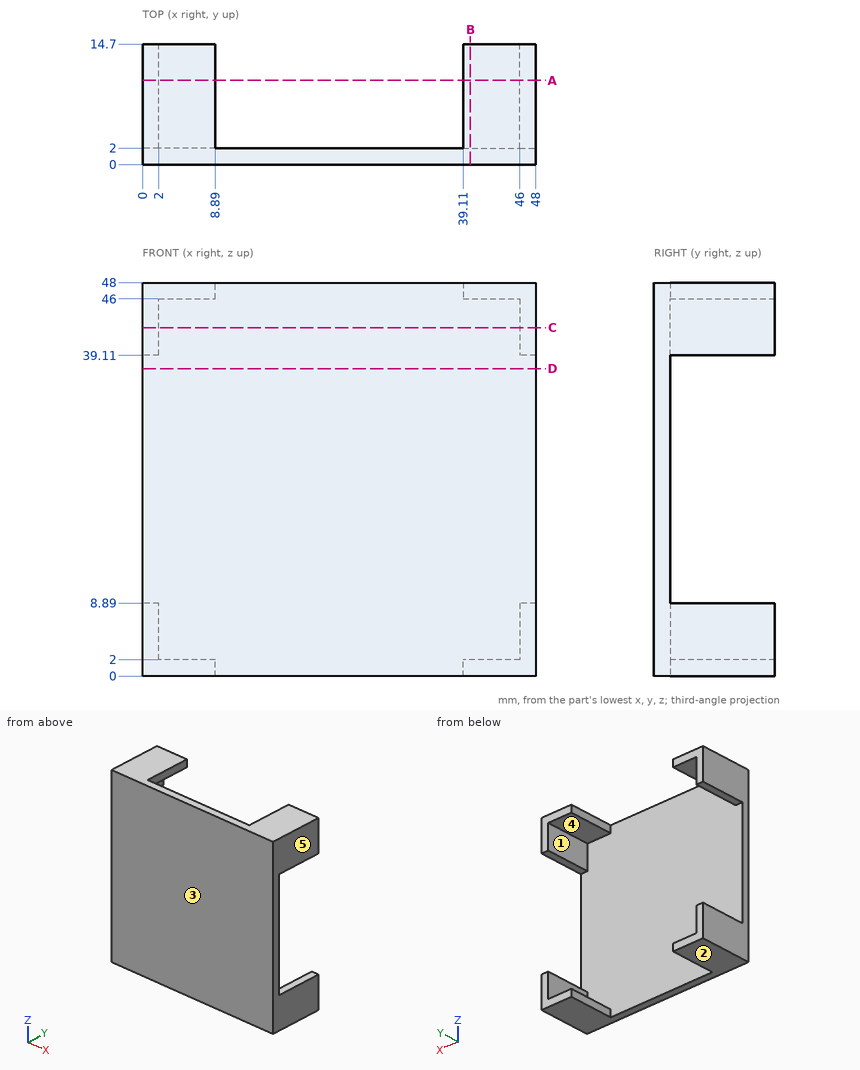
For this review, use the dimensioned drawing (mm, ordinates from the lowest corner) and the shaded views. A direction names the side the tool comes from. Coordinates: 2 decimals unless noted, no trailing zeros. Write each loop counter-clockwise with the first axis right and the second up, starting at its lowest first coordinate (ties: lowest second). Pieces come first, ordered by that corner, then holes. Notation, with made-up numbers: (-12.5, 49.25) - (45.5, 49.25) arc R18 ccw to (45.5, 55.25) - close; hole circle Ø5 at (3, 81). An arc over 180 degrees is marked (long way). One line per item, written item: value.
1) Add section B-B (x = 40). State the section outline as (y, z) points, plus the area to 3 significant figures.
Answer sheet:
outline: (0, 0) - (14.7, 0) - (14.7, 2) - (2, 2) - (2, 46) - (14.7, 46) - (14.7, 48) - (0, 48) - close
area: 147 mm2
2) Add section D-D (z = 37.5). State the section outline as (x, y) points.
Answer sheet:
outline: (0, 0) - (48, 0) - (48, 2) - (0, 2) - close
3) Add section C-C (z = 42.5). State the section outline as (x, y) points.
Answer sheet:
outline: (0, 0) - (48, 0) - (48, 14.7) - (46, 14.7) - (46, 2) - (2, 2) - (2, 14.7) - (0, 14.7) - close
4) For the marked faces 4 and 5, list the 3-axis set-ups (+Z, -Z, +X, -X, +Y, -Y) from which the entire face can be reached by the end or side of a thin tool; tool diameter is ignored.
Answer sheet:
face 4: +Y
face 5: +Z, -Z, +X, +Y, -Y
5) Mouldability with a two-part tool opening along Z and no side actions: class the marked faces 1, 2 and 3 as +Z half, -Z half, draft (parallel to the pull), parting line (faces both ways), or undercut.
Answer sheet:
face 1: undercut
face 2: -Z half
face 3: draft
6) To check wall thickness, follow probe 1 along X at (y, z) = (5.75, 5.5); probe 2 along Y at (x, z) = (8, 35). State the ranges of each line that lie inside material, in increasing order.
Answer sheet:
probe 1: x = 0 to 2, 46 to 48
probe 2: y = 0 to 2
7) Insertion check: pin 1 (7.5 mm diameter, centred on x = 4.5, y = 7, fed in from -Z); pin 2 (1.5 mm diameter, centred on x = 6, z = 35, fed in from +Y). Each pin has a flat end and moves straight along its axis. Give the tip position at first contact, or say it passes through.
Answer sheet:
pin 1: stops at z = 0
pin 2: stops at y = 2
8) Add section A-A (y = 10.25). State the section outline as (x, z) points.
Answer sheet:
outline: (0, 0) - (8.89, 0) - (8.89, 2) - (2, 2) - (2, 8.89) - (0, 8.89) - close; (0, 39.11) - (2, 39.11) - (2, 46) - (8.89, 46) - (8.89, 48) - (0, 48) - close; (39.11, 0) - (48, 0) - (48, 8.89) - (46, 8.89) - (46, 2) - (39.11, 2) - close; (39.11, 46) - (46, 46) - (46, 39.11) - (48, 39.11) - (48, 48) - (39.11, 48) - close
